For this review, take the finished solid that the model builds, in its own axes (mm). Face numbers are marked on the shaded views. A direction names the side the tool comes from. Round coordinates to 2 decimals unless told otherwise and drop trailing zeros. Loops run counter-clockwise (first coordinate to the right, second up) from the corner with the lowest first, then second, coordinate; pieces in that order, holes last.
```python
from build123d import *

# Parameters (mm, degrees)
CYLINDER219_R          = 1.7
CYLINDER219_DEPTH      = 20
CYLINDER219_ROLL_ANGLE = 90
CYLINDER218_R          = 1.7
CYLINDER218_DEPTH      = 20
CYLINDER218_ROLL_ANGLE = 90
CYLINDER217_R          = 4.2
CYLINDER217_DEPTH      = 18
CYLINDER217_ROLL_ANGLE = 90
BOX001027045165_W      = 10
BOX001027045165_H      = 4
BOX001027045165_DEPTH  = 60
CYLINDER216_R          = 2
CYLINDER216_DEPTH      = 74
BOX001027045155_W      = 16
BOX001027045155_H      = 4.5
BOX001027045155_DEPTH  = 12
FILLET032_R            = 7


with BuildPart() as cylinder258:
    # Cylinder219 → Cylinder219 (new body)
    with BuildSketch(Plane.XY):
        Circle(CYLINDER219_R)
    extrude(amount=CYLINDER219_DEPTH)


with BuildPart() as cylinder258_1:
    # Cylinder219 roll: moved
    add(cylinder258.part.rotate(Axis((0, 0, 0), (1, 0, 0)), CYLINDER219_ROLL_ANGLE))


with BuildPart() as cylinder258_2:
    # Cylinder219 placement: moved
    add(cylinder258_1.part.moved(Location((7, 11, -13))))


with BuildPart() as top_slot_m3_clearance:
    # Cylinder218 → Cylinder218 (new body)
    with BuildSketch(Plane.XY):
        Circle(CYLINDER218_R)
    extrude(amount=CYLINDER218_DEPTH)


with BuildPart() as top_slot_m3_clearance_1:
    # Cylinder218 roll: moved
    add(top_slot_m3_clearance.part.rotate(Axis((0, 0, 0), (1, 0, 0)), CYLINDER218_ROLL_ANGLE))


with BuildPart() as top_slot_m3_clearance_2:
    # Cylinder218 placement: moved
    add(top_slot_m3_clearance_1.part.moved(Location((7, 11, -19))))

    # Fusion112117: union Cylinder258
    add(cylinder258_2.part)


with BuildPart() as rocker_cut002:
    # Cylinder217 → Cylinder217 (new body)
    with BuildSketch(Plane.XY):
        Circle(CYLINDER217_R)
    extrude(amount=CYLINDER217_DEPTH)


with BuildPart() as rocker_cut002_1:
    # Cylinder217 roll: moved
    add(rocker_cut002.part.rotate(Axis((0, 0, 0), (1, 0, 0)), CYLINDER217_ROLL_ANGLE))


with BuildPart() as rocker_cut002_2:
    # Cylinder217 placement: moved
    add(rocker_cut002_1.part.moved(Location((0, 9, -8))))


with BuildPart() as cube213:
    # Box001027045165 → Box001027045165 (new body)
    with BuildSketch(Plane(origin=(-10, -2, -57), x_dir=(1, 0, 0), z_dir=(0, 0, 1))):
        with Locations((5, 2)):
            Rectangle(BOX001027045165_W, BOX001027045165_H)
    extrude(amount=BOX001027045165_DEPTH)


with BuildPart() as fusion112116:
    # Cylinder216 → Cylinder216 (new body)
    with BuildSketch(Plane.XY.offset(-62)):
        Circle(CYLINDER216_R)
    extrude(amount=CYLINDER216_DEPTH)

    # Fusion112116: union Cube213
    add(cube213.part)


with BuildPart() as fusion112116_1:
    # Fusion112116 placement: moved
    add(fusion112116.part.moved(Location((2.5, 0, 0))))


with BuildPart() as top_slot_plate:
    # Box001027045155 → Box001027045155 (new body)
    with BuildSketch(Plane(origin=(-5, 0, -22), x_dir=(1, 0, 0), z_dir=(0, 0, 1))):
        with Locations((8, 2.25)):
            Rectangle(BOX001027045155_W, BOX001027045155_H)
    extrude(amount=BOX001027045155_DEPTH)

    # Cut196: cut Fusion112116
    add(fusion112116_1.part, mode=Mode.SUBTRACT)

    # Cut197: cut rocker-cut002
    add(rocker_cut002_2.part, mode=Mode.SUBTRACT)

    # Cut198: cut top-slot-m3-clearance
    add(top_slot_m3_clearance_2.part, mode=Mode.SUBTRACT)

    # Fillet032
    fillet032_edges = [top_slot_plate.edges().sort_by_distance(p)[0] for p in [
        (-5, 3.25, -22),
    ]]
    fillet(fillet032_edges, radius=FILLET032_R)


solid = top_slot_plate.part
```
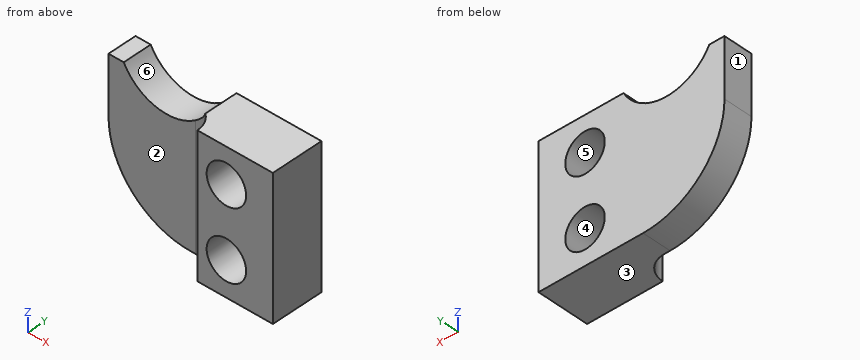
(1) Insertion check: pin 1 Ø2.5 at (x, z) = (7, -19) entering from -Y; pin 2 Ø1.5 at (y, z) = (2, -18.5) entering from -X. Each pin has a flat end and moves straight along its axis. Give the tip position at first contact, or say it passes through.
(2) For L1, parallel to Z at x = 7, y = 2.15; L2, parallel to X at y = 2.4, z = -13; L3, parallel to Z at x = 5.5, y = 1.45, list the stretches that pass through material, from the lowest coordinate up.
(3) Add section C-C (x = 7). Give the boundary of the cut face in (y, z).
(4) For the marked faces 1 and 2, list the 3-axis set-ups (+Z, -Z, +X, -X, +Y, -Y) from which the entire face can be reached by the end or side of a thin tool; tool diameter is ignored.
(5) Add section A-A (z = -13). Give the boundary of the cut face in (x, y).
(6) The part is to be moulded in two halves that separate along Z. For the marked faces 3, 4, 5 and 6, say which applies: pulls with the +Z half, pulls with the -Z half, needs draft (parallel to the pull), parting line crosses it, or undercut.
(7) Add section B-B (y = 3.85). Give the boundary of the cut face in (x, z).
(8) Add section D-D (z = -11.75). Give the boundary of the cut face in (x, y), plus the area to 3 significant figures.
Outcome:
1. pin 1: passes through
1. pin 2: stops at x = -4.44
2. L1: z = -22 to -20.7, -17.3 to -14.7, -11.3 to -10
2. L2: x = -5 to 5.3, 8.7 to 11
2. L3: z = -22 to -19.8, -18.2 to -13.8, -12.2 to -10
3. outline: (0, -22) - (4.5, -22) - (4.5, -20.7) - (0, -20.7) - close; (0, -17.3) - (4.5, -17.3) - (4.5, -14.7) - (0, -14.7) - close; (0, -11.3) - (4.5, -11.3) - (4.5, -10) - (0, -10) - close
4. face 1: +Z, -Z, -X, +Y, -Y
4. face 2: +Z, -Z, -X, -Y
5. outline: (-5, 2) - (2.5, 2) arc R2 cw to (4.5, 0) - (5.3, 0) - (5.3, 4.5) - (-5, 4.5) - close; (8.7, 0) - (11, 0) - (11, 4.5) - (8.7, 4.5) - close
6. face 3: pulls with the -Z half
6. face 4: undercut
6. face 5: undercut
6. face 6: pulls with the +Z half
7. outline: (-5, -15) arc R7 ccw to (2, -22) - (11, -22) - (11, -10) - (3.69, -10) arc R4.2 cw to (-3.69, -10) - (-5, -10) - close; hole circle Ø3.4 at (7, -19); hole circle Ø3.4 at (7, -13)
8. outline: (-5, 2) - (-1.89, 2) - (-1.89, 4.5) - (-5, 4.5) - close; (1.89, 2) - (2.5, 2) arc R2 cw to (4.5, 0) - (5.85, 0) - (5.85, 4.5) - (1.89, 4.5) - close; (8.15, 0) - (11, 0) - (11, 4.5) - (8.15, 4.5) - close
8. area: 34.0 mm2
